Verification items for this drawing (mm, ordinates from the low corner). A direction names the side the tool comes from. Round coordinates to 2 decimals unless told otherwise and drop trailing zeros. Write each loop counter-clockwise with the first axis right and the second up, starting at its lowest first coordinate (ties: lowest second). Pieces come first, ordered by that corner, then holes. Notation, with made-up numbers: (-33, -20.5) -> (7, -20.5) arc R13 ccw to (7, -3.5) -> close; hole circle Ø10 at (-12, 58.25). An arc over 180 degrees is marked (long way). Return JSON: item names as keys, results as strings. Group by question number.
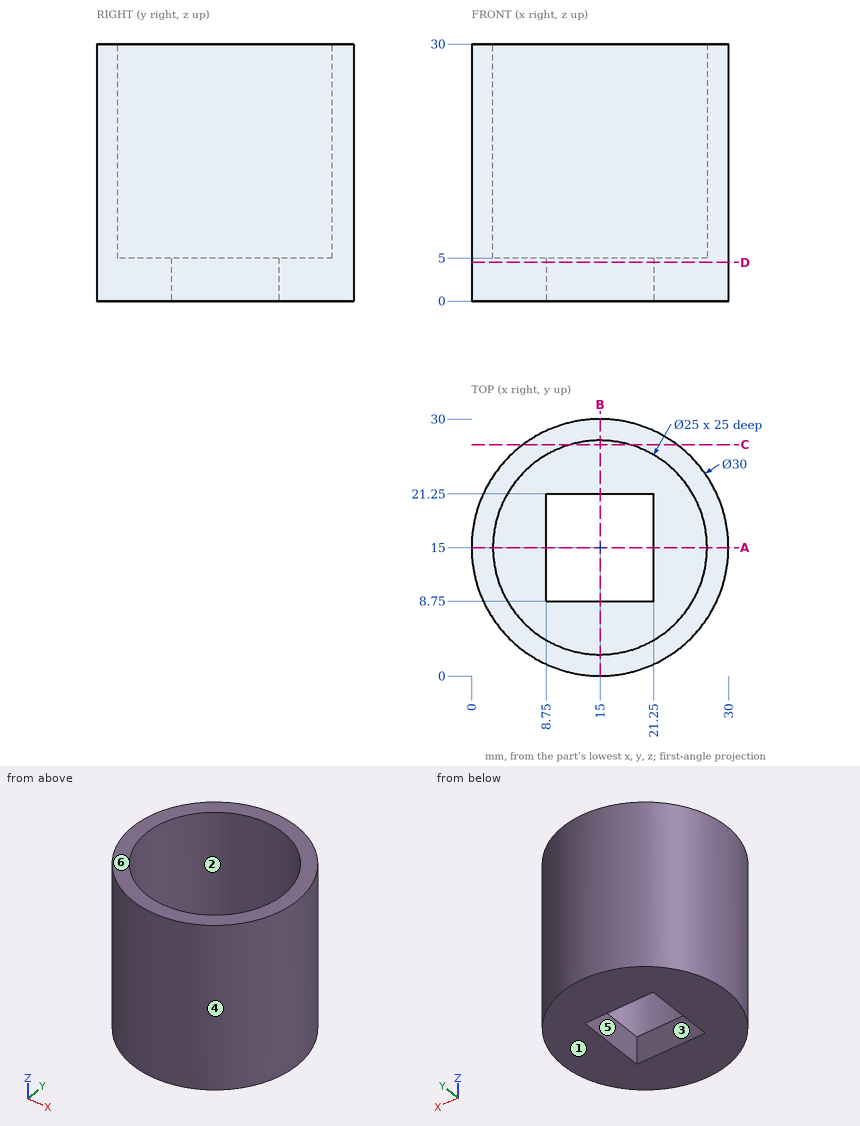
1) Sectioned sample at A-A on y = 15. Enter the section's corners in (x, z).
2) Mould release check, pull along Y, two halves, no side actions. Record for the marked faces 1, 2, 3 and 4: +Y half, -Y half, draft (parallel to the pull), parting line (faces both ways), or undercut.
3) Sectioned sample at C-C on y = 27. Enter the section's corners in (x, z).
4) Go/stop test with flat-tipped pins: P1, Ø2, axis at x = 23.5, z = 16, coming from the +Y side; P2, Ø1, axis at x = 25, z = 23.5, coming from the -Y side; P3, Ø5.5, axis at x = 16, z = 1.5, coming from the +Y side; P4, Ø8, axis at y = 8, z = 25.5, coming from the -X side. Record where each tip stops, or that it passes through.
5) Tool access check on the marked faces 5 and 6. Record the directions out of +Z, -Z, +X, -X, +Y, -Y that give a thin tool (end or side, any length) a straight path to the whole face; none if there is none.
6) Material ranges on probe 1 along Y at (x, z) = (15, 8.5); probe 2 along Z at (x, y) = (6.5, 21.75); probe 3 along Y at (x, z) = (22.25, 6.75), recorded low to high. Write a range as [from, to].
7) Sectioned sample at D-D on z = 4.5. Enter the section's corners in (x, y).
Evaluation:
{
 "1": {"outline": "(0, 0) -> (8.75, 0) -> (8.75, 5) -> (2.5, 5) -> (2.5, 30) -> (0, 30) -> close; (21.25, 0) -> (30, 0) -> (30, 30) -> (27.5, 30) -> (27.5, 5) -> (21.25, 5) -> close"},
 "2": {"face 1": "draft", "face 2": "undercut", "face 3": "undercut", "face 4": "parting line"},
 "3": {"outline": "(6, 0) -> (24, 0) -> (24, 30) -> (18.5, 30) -> (18.5, 5) -> (11.5, 5) -> (11.5, 30) -> (6, 30) -> close"},
 "4": {"P1": "stops at y = 27.99", "P2": "stops at y = 3.39", "P3": "stops at y = 30", "P4": "stops at x = 0.3"},
 "5": {"face 5": "+Z, -Z", "face 6": "+Z, +X, -X, +Y, -Y"},
 "6": {"probe 1": "y = [0, 2.5], [27.5, 30]", "probe 2": "z = [0, 5]", "probe 3": "y = [1.87, 4.82], [25.18, 28.13]"},
 "7": {"outline": "circle Ø30 at (15, 15); hole (8.75, 8.75) -> (21.25, 8.75) -> (21.25, 21.25) -> (8.75, 21.25) -> close"}
}
